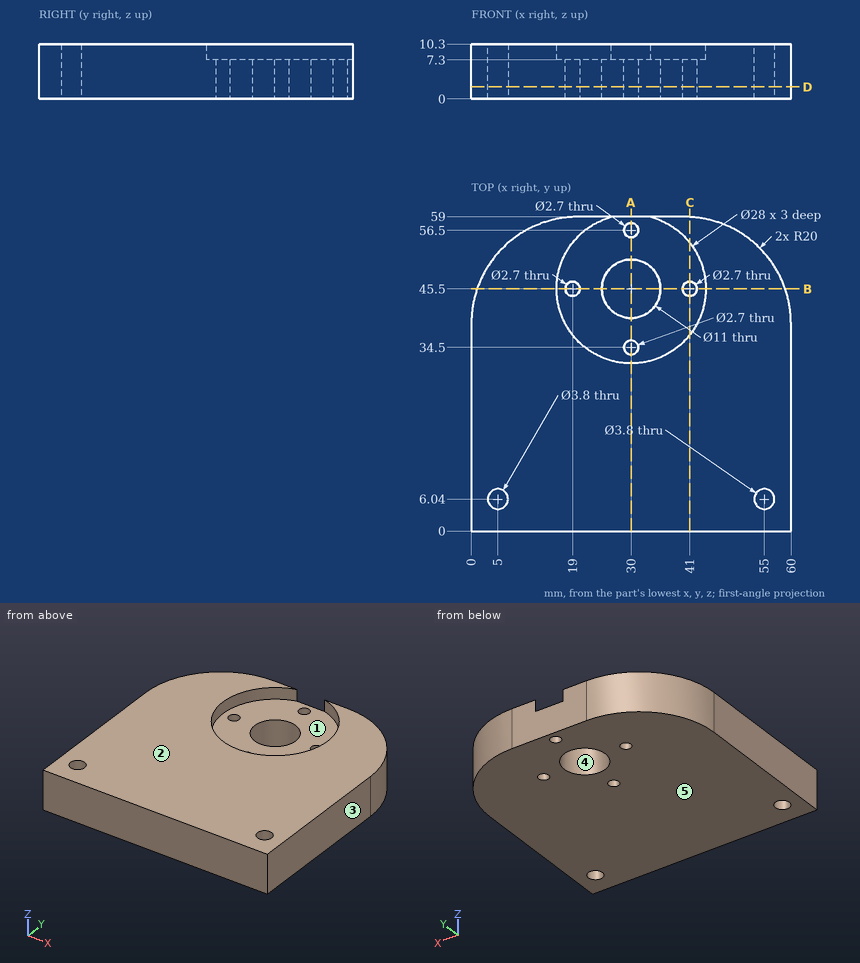
The drawing under review shows one solid part. Ordinate dimensions are in mm from its lowest x, y, z. A direction names the side the tool comes from. Coordinates: 2 decimals unless noted, no trailing zeros. Write each loop counter-clockwise with the first axis right and the second up, starting at its lowest first coordinate (ties: lowest second). Pieces come first, ordered by that corner, then holes. Notation, with made-up numbers: (28.5, 60.25) - (81.5, 60.25) arc R21 ccw to (81.5, 98.25) - close; hole circle Ø1 at (-5.75, 3.25). An arc over 180 degrees is marked (long way). Put each result on its own line as item: value.
1. Add section D-D, the plane z = 2.25. Give the boundary of the cut face in (x, y).
Values found:
outline: (0, 0) - (60, 0) - (60, 39) arc R20 ccw to (40, 59) - (20, 59) arc R20 ccw to (0, 39) - close; hole circle Ø3.8 at (5, 6.04); hole circle Ø2.7 at (19, 45.5); hole circle Ø11 at (30, 45.5); hole circle Ø2.7 at (30, 34.5); hole circle Ø2.7 at (30, 56.5); hole circle Ø2.7 at (41, 45.5); hole circle Ø3.8 at (55, 6.04)
2. Machinability: for the marked faces 1 and 2, which of the approach directions +Z, -Z, +X, -X, +Y, -Y give a long, thin tool a straight path to every point of the face, cutting with its end or side? Answer none if there is none.
Values found:
face 1: +Z
face 2: +Z, +X, -X, +Y, -Y
3. Mouldability with a two-part tool opening along X and no side actions: class the marked faces 3, 4 and 5 as released by +X, released by -X, zero draft, split by the parting line, or undercut.
Values found:
face 3: released by +X
face 4: undercut
face 5: zero draft
4. Add section C-C, the plane x = 41. Give the boundary of the cut face in (y, z), then the cut area to 3 significant figures.
Values found:
outline: (0, 0) - (44.15, 0) - (44.15, 7.3) - (36.84, 7.3) - (36.84, 10.3) - (0, 10.3) - close; (46.85, 0) - (58.97, 0) - (58.97, 10.3) - (54.16, 10.3) - (54.16, 7.3) - (46.85, 7.3) - close
area: 536 mm²
5. Add section A-A, the plane x = 30. Give the boundary of the cut face in (y, z).
Values found:
outline: (0, 0) - (33.15, 0) - (33.15, 7.3) - (31.5, 7.3) - (31.5, 10.3) - (0, 10.3) - close; (35.85, 0) - (40, 0) - (40, 7.3) - (35.85, 7.3) - close; (51, 0) - (55.15, 0) - (55.15, 7.3) - (51, 7.3) - close; (57.85, 0) - (59, 0) - (59, 7.3) - (57.85, 7.3) - close
6. Wall thickness on probe 1 along Y at (x, z) = (30, 5.5); probe 2 along X at (y, z) = (34.5, 3.75); probe 3 along X at (y, z) = (6, 3.25): over which ranges is each line inside the solid? List them lowest first.
Values found:
probe 1: 0 to 33.15, 35.85 to 40, 51 to 55.15, 57.85 to 59
probe 2: 0 to 28.65, 31.35 to 60
probe 3: 0 to 3.1, 6.9 to 53.1, 56.9 to 60
7. Add section B-B, the plane y = 45.5. Give the boundary of the cut face in (x, z), then the cut area to 3 significant figures.
Values found:
outline: (1.09, 0) - (17.65, 0) - (17.65, 7.3) - (16, 7.3) - (16, 10.3) - (1.09, 10.3) - close; (20.35, 0) - (24.5, 0) - (24.5, 7.3) - (20.35, 7.3) - close; (35.5, 0) - (39.65, 0) - (39.65, 7.3) - (35.5, 7.3) - close; (42.35, 0) - (58.91, 0) - (58.91, 10.3) - (44, 10.3) - (44, 7.3) - (42.35, 7.3) - close
area: 392 mm²
8. For pin 1 (14 mm diameter, centred on x = 31, y = 50.5, fed in from +Z); pin 2 (25 mm diameter, centred on x = 30, y = 45.5, fed in from -Z), all flat-tipped, find the tip position at first contact; note any pin that passes through.
Values found:
pin 1: z = 7.3
pin 2: z = 0
